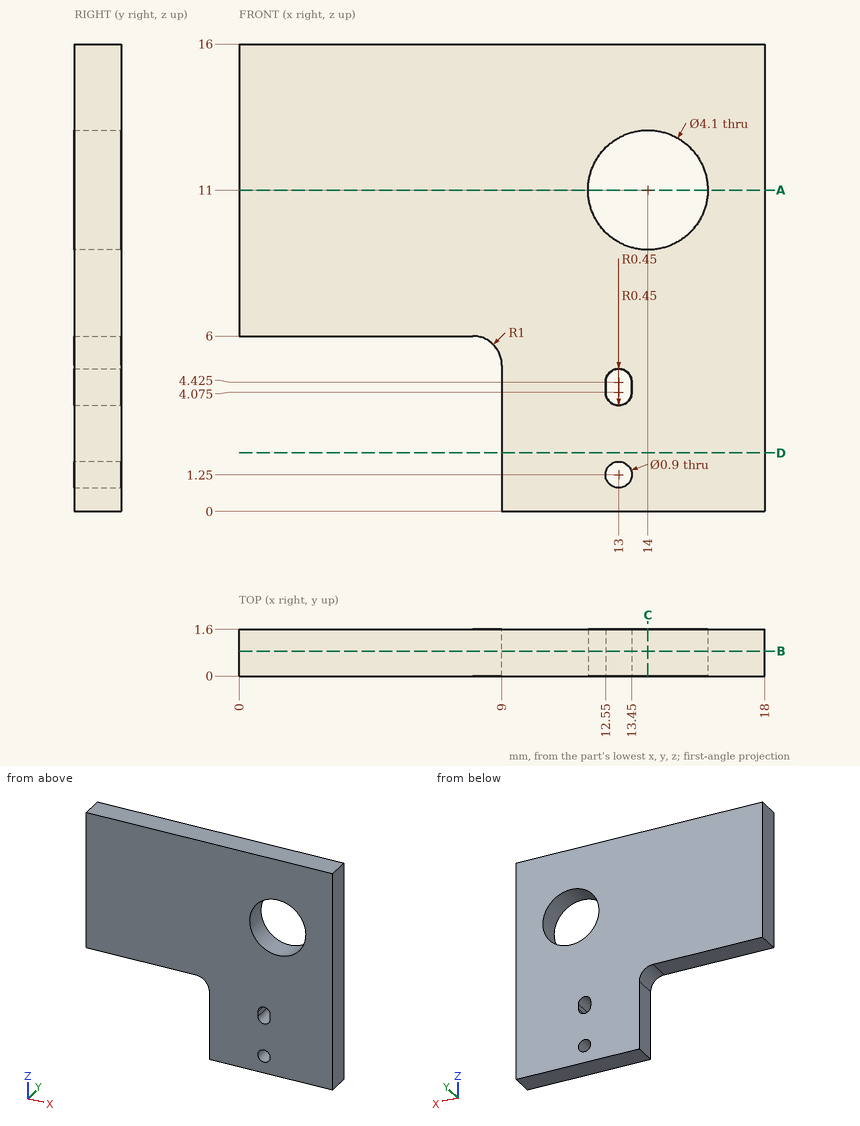
Answer from the drawing. Dimensions are ordinates in mm from the lowest x, y and z of the part. Give positions to 0.01 mm unless a question says otherwise; leave off trailing zeros. Loops run counter-clockwise (first coordinate to the right, second up) from the corner with the lowest first, then second, coordinate; pieces in that order, holes last.
Item 1: Each of these flat-tipped pins is pushed along its axis until it touches: pin 1 Ø2 at (x, z) = (2.5, 10.5) entering from -Y; pin 2 Ø0.8 at (x, y) = (2, 1) entering from -Z. Where does it stop, or does it pass through?
Item 2: The part is cut by section D-D (z = 2). Write down the section's boundary in (x, y), and give its area (3 significant figures).
Item 3: Find the intervals of material crossed by line 1 along X through (y, z) = (0.5, 11); line 2 along X through (y, z) = (0.85, 1.25); line 3 along Z through (x, y) = (7.5, 1), in increasing order.
Item 4: The part is cut by section C-C (x = 14). Write down the section's boundary in (y, z), and give its area (3 significant figures).
Item 5: The part is cut by section A-A (z = 11). Write down the section's boundary in (x, y), and give its area (3 significant figures).
Item 6: The part is cut by section B-B (y = 0.85). Write down the section's boundary in (x, z) (3 decimals).
Taken from the geometry:
1. pin 1: stops at y = 0
1. pin 2: stops at z = 6
2. outline: (9, 0) - (18, 0) - (18, 1.6) - (9, 1.6) - close
2. area: 14.4 mm2
3. line 1: x = 0 to 11.95, 16.05 to 18
3. line 2: x = 9 to 12.55, 13.45 to 18
3. line 3: z = 6 to 16
4. outline: (0, 0) - (1.6, 0) - (1.6, 8.95) - (0, 8.95) - close; (0, 13.05) - (1.6, 13.05) - (1.6, 16) - (0, 16) - close
4. area: 19.0 mm2
5. outline: (0, 0) - (11.95, 0) - (11.95, 1.6) - (0, 1.6) - close; (16.05, 0) - (18, 0) - (18, 1.6) - (16.05, 1.6) - close
5. area: 22.2 mm2
6. outline: (0, 6) - (8, 6) arc R1 cw to (9, 5) - (9, 0) - (18, 0) - (18, 16) - (0, 16) - close; hole circle Ø4.1 at (14, 11); hole circle Ø0.9 at (13, 1.25); hole (12.55, 4.075) arc R0.45 ccw to (13.45, 4.075) - (13.45, 4.425) arc R0.45 ccw to (12.55, 4.425) - close
